Model file for the job. Use its own axes, mm. Give positions to 0.01 mm unless a question says otherwise; leave off trailing zeros. Use CSV: the item, a comma, the result in double quotes. Start each with the question number.
(1) Flat gauge pins, fed straight in: pin 1 (1.4 mm diameter, centred on x = 1, z = 209, fed in from +Y); pin 2 (1 mm diameter, centred on x = -3.5, y = -5.5, fed in from -Z); pin 3 (1 mm diameter, centred on y = -2.5, z = 470.5, fed in from -X); pin 4 (1.4 mm diameter, centred on x = 0.5, z = 453, fed in from -Y). Where does each tip first touch, or does it go through?
(2) Pull direction Y, two halves, no side cores. Call faces 1 (the flat face through (4, 0, 0)), 2 (the flat face through (10, 20, 316)), 3 (the flat face through (-10, -20, 316)): pulls with the +Y half, pulls with the -Y half, needs draft (parallel to the pull), parting line crosses it, or undercut.
(3) Drill centre lines: probe 1 along Y at (x, z) = (-17, 459.5); probe 2 along Y at (x, z) = (0, 247); probe 3 along X at (y, z) = (-11, 393.5). Where is each one in solid material? Low to high.
Autodesk Inventor part; units mm, degrees
ref_plane "YZ Plane" through (0, 0, 0) normal (1, 0, 0) x (0, 1, 0)
ref_plane "XZ Plane" through (0, 0, 0) normal (0, 1, 0) x (-1, 0, 0)
ref_plane "XY Plane" through (0, 0, 0) normal (0, 0, 1) x (1, 0, 0)
sketch "T-Slot 4040 Base" plane through (0, 0, 0) normal (0, 0, 1) x (1, 0, 0)
  line L0 (-28, 0) -> (28, 0) construction
  line L1 (0, -28) -> (0, 28) construction
  circle A0 centre (0, 0) radius 3.4
  line L2 (-7.5, -7.5) -> (7.5, -7.5)
  line L3 (7.5, -7.5) -> (7.5, 7.5)
  line L4 (7.5, 7.5) -> (-7.5, 7.5)
  line L5 (-7.5, 7.5) -> (-7.5, -7.5)
  line L6 (-7.5, -7.5) -> (7.5, 7.5) construction
  line L7 (7.5, -7.5) -> (-7.5, 7.5) construction
  line L8 (20, 4) -> (15.5, 4)
  line L9 (15.5, 4) -> (15.5, 12)
  line L10 (15.5, 12) -> (7.5, 4)
  line L11 (4, 20) -> (4, 15.5)
  line L12 (4, 15.5) -> (12, 15.5)
  line L13 (12, 15.5) -> (4, 7.5)
  line L14 (7.5, -7.5) -> (-7.5, -7.5)
  arc A1 (15.5, 9.5858) -> (13.7929, 10.2929) centre (14.5, 9.5858) ccw
  arc A2 (10.2929, 13.7929) -> (9.5858, 15.5) centre (9.5858, 14.5) ccw
  line L15 (-20, 20) -> (20, 20)
  line L16 (20, 20) -> (20, -20)
  line L17 (20, -20) -> (-20, -20)
  line L18 (-20, -20) -> (-20, 20)
  line L19 (-20, 20) -> (20, -20) construction
  line L20 (20, 20) -> (-20, -20) construction
  line L21 (-4, 15.5) -> (-12, 15.5)
  arc A3 (-9.5858, 15.5) -> (-10.2929, 13.7929) centre (-9.5858, 14.5) ccw
  line L22 (-12, 15.5) -> (-4, 7.5)
  line L23 (-15.5, 12) -> (-7.5, 4)
  line L24 (-20, 4) -> (-15.5, 4)
  arc A4 (-13.7929, 10.2929) -> (-15.5, 9.5858) centre (-14.5, 9.5858) ccw
  line L25 (-15.5, 4) -> (-15.5, 12)
  line L26 (-4, 20) -> (-4, 15.5)
  line L27 (-15.5, -4) -> (-15.5, -12)
  arc A5 (-15.5, -9.5858) -> (-13.7929, -10.2929) centre (-14.5, -9.5858) ccw
  line L28 (-15.5, -12) -> (-7.5, -4)
  line L29 (-12, -15.5) -> (-4, -7.5)
  line L30 (-4, -20) -> (-4, -15.5)
  arc A6 (-10.2929, -13.7929) -> (-9.5858, -15.5) centre (-9.5858, -14.5) ccw
  line L31 (-4, -15.5) -> (-12, -15.5)
  line L32 (-20, -4) -> (-15.5, -4)
  line L33 (4, -15.5) -> (12, -15.5)
  arc A7 (9.5858, -15.5) -> (10.2929, -13.7929) centre (9.5858, -14.5) ccw
  line L34 (12, -15.5) -> (4, -7.5)
  line L35 (15.5, -12) -> (7.5, -4)
  line L36 (20, -4) -> (15.5, -4)
  arc A8 (13.7929, -10.2929) -> (15.5, -9.5858) centre (14.5, -9.5858) ccw
  line L37 (15.5, -4) -> (15.5, -12)
  line L38 (4, -20) -> (4, -15.5)
  point P0 (4.9274, 7.75)
  point P1 (9.5858, 15.5)
  point P2 (-20, 20)
  point P3 (-7.5, -7.5)
  point P4 (-20, -20)
  point P5 (7.5, -7.5)
  point P6 (20, -20)
  point P7 (-9.5858, -15.5)
  point P8 (-4, -7.5)
  point P9 (15.5, -9.5858)
  point P10 (7.5, -4)
  point P11 (-15.5, 9.5858)
  point P12 (-4, 7.5)
  dimension "d35" = 6.8
  dimension "d37" = 12
  dimension "d38" = 1
  dimension "d43" = 40
  dimension "d44" = 40
  dimension "d45" = 4.5
  dimension "d46" = 4
  dimension "d53" = 360
extrude "Extrusion1" add sketch "T-Slot 4040 Base" along normal blind 640 contours L5 L4 L3 L2 | L2 L29 L31 L30 L17 L18 L32 L27 L28 L5 | L2 L3 L35 L37 L36 L16 L17 L38 L33 L34 | A6 L31 L29 | L23 L25 L24 L18 L15 L26 L21 L22 L4 L5 | L28 L27 A5 | L34 L33 A7 | A4 L25 L23 | L3 L4 L13 L12 L11 L15 L16 L8 L9 L10 | A8 L37 L35 | L22 L21 A3 | L10 L9 A1 | A2 L12 L13
fillet "Rundung1" radius 1 16 edges at (4, 15.5, 320) (15.5, 4, 320) (20, 4, 320) (4, 20, 320) (-20, 4, 320) (-15.5, 4, 320) (-4, 15.5, 320) (-4, 20, 320) (-4, -15.5, 320) (-4, -20, 320) (4, -15.5, 320) (4, -20, 320) (15.5, -4, 320) (20, -4, 320) (-20, -4, 320) (-15.5, -4, 320)
fillet "Rundung2" radius 4 12 edges at (4, 7.5, 320) (7.5, 4, 320) (-20, 20, 320) (-20, -20, 320) (20, 20, 320) (20, -20, 320) (7.5, -4, 320) (-7.5, -4, 320) (-7.5, 4, 320) (4, -7.5, 320) (-4, -7.5, 320) (-4, 7.5, 320)
properties part number "T-SLOT 4040 B-Type 640mm"
Check result:
1,pin 1,"y = 7.5"
1,pin 2,"z = 0"
1,pin 3,"x = -7.55"
1,pin 4,"y = -7.5"
2,face 1,"needs draft"
2,face 2,"pulls with the +Y half"
2,face 3,"pulls with the -Y half"
3,probe 1,"-19.87 to -4, 4 to 19.87"
3,probe 2,"-7.5 to -3.4, 3.4 to 7.5"
3,probe 3,"-20 to -7.5, 7.5 to 20"
